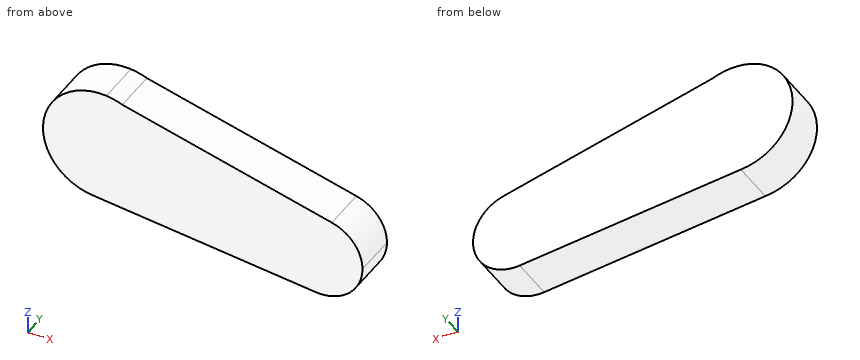
from build123d import *

# Parameters (mm, degrees)
F1_DEPTH = 25.4
F2_DEPTH = 25.4


with BuildPart() as f1:
    # F0 (on Front) → F1 (new body)
    with BuildSketch(Plane.XZ):
        with BuildLine():
            Line((-50.770752, 68.621059), (-59.689327, 71.015835))
            ThreePointArc((-59.689327, 71.015835), (-94.933334, 42.775326), (-66.24222, 7.897161))
            ThreePointArc((-66.24222, 7.897161), (-41.972825, 16.067976), (-31.63981, 39.498609))
            ThreePointArc((-31.63981, 39.498609), (-36.850348, 56.920649), (-50.770752, 68.621059))
        make_face()
        with BuildLine():
            ThreePointArc((-50.770752, 68.621059), (-55.142458, 70.144617), (-59.689327, 71.015835))
            Line((-59.689327, 71.015835), (-50.770752, 68.621059))
        make_face()
        with BuildLine():
            ThreePointArc((-31.63981, 39.498609), (-41.972825, 16.067976), (-66.24222, 7.897161))
            Line((-66.24222, 7.897161), (57.235367, -8.014038))
            ThreePointArc((57.235367, -8.014038), (37.521425, 19.385006), (66.180401, 37.217846))
            Line((66.180401, 37.217846), (-50.770752, 68.621059))
            ThreePointArc((-50.770752, 68.621059), (-36.850348, 56.920649), (-31.63981, 39.498609))
        make_face()
        with BuildLine():
            ThreePointArc((66.180401, 37.217846), (37.521425, 19.385006), (57.235367, -8.014038))
            ThreePointArc((57.235367, -8.014038), (75.446993, -2.448604), (83.294276, 14.902405))
            ThreePointArc((83.294276, 14.902405), (78.523231, 28.963554), (66.180401, 37.217846))
        make_face()
    extrude(amount=F1_DEPTH)

    # F0 (on Front) → F2 (join)
    with BuildSketch(Plane.XZ):
        with BuildLine():
            Line((-50.770752, 68.621059), (-59.689327, 71.015835))
            ThreePointArc((-59.689327, 71.015835), (-94.933334, 42.775326), (-66.24222, 7.897161))
            ThreePointArc((-66.24222, 7.897161), (-41.972825, 16.067976), (-31.63981, 39.498609))
            ThreePointArc((-31.63981, 39.498609), (-36.850348, 56.920649), (-50.770752, 68.621059))
        make_face()
        with BuildLine():
            ThreePointArc((-50.770752, 68.621059), (-55.142458, 70.144617), (-59.689327, 71.015835))
            Line((-59.689327, 71.015835), (-50.770752, 68.621059))
        make_face()
        with BuildLine():
            ThreePointArc((-31.63981, 39.498609), (-41.972825, 16.067976), (-66.24222, 7.897161))
            Line((-66.24222, 7.897161), (57.235367, -8.014038))
            ThreePointArc((57.235367, -8.014038), (37.521425, 19.385006), (66.180401, 37.217846))
            Line((66.180401, 37.217846), (-50.770752, 68.621059))
            ThreePointArc((-50.770752, 68.621059), (-36.850348, 56.920649), (-31.63981, 39.498609))
        make_face()
        with BuildLine():
            ThreePointArc((66.180401, 37.217846), (37.521425, 19.385006), (57.235367, -8.014038))
            ThreePointArc((57.235367, -8.014038), (75.446993, -2.448604), (83.294276, 14.902405))
            ThreePointArc((83.294276, 14.902405), (78.523231, 28.963554), (66.180401, 37.217846))
        make_face()
    extrude(amount=F2_DEPTH)


solid = f1.part
Work out the finished part from the listing and answer in its coordinate system (mm). Round coordinates to 2 decimals unless told otherwise and drop trailing zeros. Order: outer loops, then holes, each group sorted by start corner. A loop starts at its lowest first (then second) coordinate and runs counter-clockwise, first axis right, second up. Notation, with made-up numbers: M 1.25,-11.75 L 16.25,-11.75 A15 ccw 16.25,11.25 Z; hole C 36,-39 d11. An arc over 180 degrees is marked long. One line per item, written item: value.
Q1. Find section B-B on x = -39. Write down the section's boundary in (y, z), then the cut area to 3 significant figures.
Derived:
outline: M -25.4,4.39 L 0,4.39 L 0,65.46 L -25.4,65.46 Z
area: 1,550 mm²
Q2. Flat-ended cylindrical pins translate along their axes: pin 1 (12 mm diameter, centred on y = -16.5, z = 56, fed in from -X); pin 2 (3 mm diameter, centred on x = -4, y = -6.5, fed in from -Z); pin 3 (8 mm diameter, centred on y = -20.5, z = 18.5, fed in from -X). Find the tip coordinate at first contact, or state that the pin passes through.
Derived:
pin 1: x = -93.31
pin 2: z = -0.32
pin 3: x = -90.17
Q3. Straight lines are drawn through the part: line 1 (X direction, y = -19.75, z = 21); line 2 (Z direction, x = 7, y = -10); line 3 (Z direction, x = 46.5, y = -3.5). For each, find the intervals that lie inside material, in ascending order.
Derived:
line 1: -89.15 to 82.48
line 2: -1.54 to 53.11
line 3: -6.63 to 42.5
Q4. Find section C-C on z = -2. Write down the section's boundary in (x, y), then the cut area to 3 significant figures.
Derived:
outline: M 10.56,-25.4 L 75.94,-25.4 L 75.94,0 L 10.56,0 Z
area: 1,660 mm²
Q5. Find section A-A on y = -21.25. Write down the section's boundary in (x, z), then the cut area to 3 significant figures.
Derived:
outline: M -66.24,7.9 L 57.24,-8.01 A23.11 ccw 83.29,14.9 A23.11 ccw 66.18,37.22 L -50.77,68.62 A31.73 ccw -59.69,71.02 A31.73 ccw long Z
area: 9,320 mm²
